from build123d import *

# Parameters (mm, degrees)
SKETCH_1_W         = 6.6
SKETCH_1_H         = 2.7
EXTRUDE_1_DEPTH    = 1.5
SKETCH_2_W         = 0.7
SKETCH_2_H         = 0.45
EXTRUDE_664_DEPTH  = 0.2
SKETCH_3_W         = 0.45
SKETCH_3_H         = 1
SKETCH_3_W_2       = 0.45404522
EXTRUDE_1058_DEPTH = 0.2
SKETCH_4_W         = 1.3
SKETCH_4_H         = 1
EXTRUDE_4_DEPTH    = 1.6
SKETCH_5_R         = 0.4
EXTRUDE_5_DEPTH    = 0.5


with BuildPart() as part:
    # 草图1 → 凸台-拉伸1 (new body)
    with BuildSketch(Plane.XY):
        Rectangle(SKETCH_1_W, SKETCH_1_H)
    extrude(amount=-EXTRUDE_1_DEPTH)

    # 草图2 → Extrude 664 (add)
    with BuildSketch(Plane.XY):
        with Locations((-3.65, 1.125)):
            Rectangle(SKETCH_2_W, SKETCH_2_H)
        with Locations((3.65, 1.125)):
            Rectangle(SKETCH_2_W, SKETCH_2_H)
        with Locations((3.65, -1.125)):
            Rectangle(SKETCH_2_W, SKETCH_2_H)
        with Locations((-3.65, -1.125)):
            Rectangle(SKETCH_2_W, SKETCH_2_H)
    extrude(amount=-EXTRUDE_664_DEPTH)

    # 草图3 → Extrude 1058 (add)
    with BuildSketch(Plane.XY):
        with Locations((2.425, -1.85)):
            Rectangle(SKETCH_3_W, SKETCH_3_H)
        with Locations((-2.425, -1.85)):
            Rectangle(SKETCH_3_W, SKETCH_3_H)
        with Locations((0.52702261, -1.85)):
            Rectangle(SKETCH_3_W_2, SKETCH_3_H)
    extrude(amount=-EXTRUDE_1058_DEPTH)

    # 草图4 → 凸台-拉伸4 (add)
    with BuildSketch(Plane(origin=(0, 1.35, 0), x_dir=(1, 0, 0), z_dir=(0, 1, 0))):
        with Locations((-0.95, 0.667693313)):
            Rectangle(SKETCH_4_W, SKETCH_4_H)
    extrude(amount=EXTRUDE_4_DEPTH)

    # 草图5 → 凸台-拉伸5 (add)
    with BuildSketch(Plane.XY):
        with Locations((1.45, -0.05)):
            Circle(SKETCH_5_R)
        with Locations((-1.55, -0.05)):
            Circle(SKETCH_5_R)
    extrude(amount=EXTRUDE_5_DEPTH)


solid = part.part
The listing builds one solid part. Answer for the finished solid, in the listing's coordinates (mm). A direction names the side the tool comes from. Give positions to 0.01 mm unless a question says otherwise; leave off trailing zeros. Loops run counter-clockwise (first coordinate to the right, second up) from the corner with the lowest first, then second, coordinate; pieces in that order, holes last. Notation, with made-up numbers: (5.5, 63.5) - (37.5, 63.5) arc R23 ccw to (37.5, 101.5) - close; hole circle Ø2 at (65.5, 13.5). An arc over 180 degrees is marked (long way). Write each question's results on one line, items separated by ' | '.
1. Consider probe 1 along Z at (x, y) = (2.75, 0.85); probe 2 along X at (y, z) = (2.65, -0.2); probe 3 along X at (y, z) = (0, -1.3). Determine where each line is inside the solid, lowest interval first. Write a range as from..to.
Resolved:
probe 1: z = -1.5..0 | probe 2: x = -1.6..-0.3 | probe 3: x = -3.3..3.3
2. Find section A-A, the plane y = -1.6. Write down the section's boundary in (x, z).
Resolved:
outline: (-2.65, -0.2) - (-2.2, -0.2) - (-2.2, 0) - (-2.65, 0) - close; (0.3, -0.2) - (0.75, -0.2) - (0.75, 0) - (0.3, 0) - close; (2.2, -0.2) - (2.65, -0.2) - (2.65, 0) - (2.2, 0) - close
3. Find section B-B, the plane z = -0.4. Write down the section's boundary in (x, y).
Resolved:
outline: (-3.3, -1.35) - (3.3, -1.35) - (3.3, 1.35) - (-0.3, 1.35) - (-0.3, 2.95) - (-1.6, 2.95) - (-1.6, 1.35) - (-3.3, 1.35) - close
4. Find section D-D, the plane x = 2.5. Write down the section's boundary in (y, z), then the cut area to 3 significant figures.
Resolved:
outline: (-2.35, -0.2) - (-1.35, -0.2) - (-1.35, -1.5) - (1.35, -1.5) - (1.35, 0) - (-2.35, 0) - close | area: 4.25 mm^2
5. Flat-ended cylindrical pins translate along their axes: P1, Ø1, axis at x = -1.5, y = 2, coming from the +Z side; P2, Ø0.7, axis at x = -0.5, y = 2.5, coming from the -Z side; P3, Ø1.2, axis at x = -1.5, z = -1, coming from the -Y side. Find the tip coordinate at first contact, or state that the pin passes through.
Resolved:
P1: stops at z = -0.17 | P2: stops at z = -1.17 | P3: stops at y = -1.35
6. Which of the six approach directions +Z, -Z, +X, -X, +Y, -Y give full straight-line access (tool end or side, diameter ignored) to faces 1 (the face through (-1, 2, -0.168)), 2 (the face through (-1.6, 2, -1)), 3 (the face through (-0.3, 2, -1))?
Resolved:
face 1: +Z, +X, -X, +Y | face 2: +Z, -Z, -X, +Y | face 3: +Z, -Z, +X, +Y
7. Find section C-C, the plane y = 1.05. Write down the section's boundary in (x, z), then the cut area to 3 significant figures.
Resolved:
outline: (-4, -0.2) - (-3.3, -0.2) - (-3.3, -1.5) - (3.3, -1.5) - (3.3, -0.2) - (4, -0.2) - (4, 0) - (-4, 0) - close | area: 10.2 mm^2
